Drawing for the job (mm, zero at the part's lowest x, y, z). A direction names the side the tool comes from. Round coordinates to 2 decimals unless told otherwise and drop trailing zeros. Write each loop counter-clockwise with the first axis right and the second up, starting at its lowest first coordinate (ties: lowest second). Pieces come first, ordered by that corner, then holes.
Item 1: Band-saw the part on D-D, the plane z = 36. Write the cut outline in (x, y).
Item 2: Band-saw the part on B-B, the plane z = 9. Write the cut outline in (x, y).
Item 3: Band-saw the part on C-C, the plane y = 2.5. Count the separate pieces of the cut face and the enclosed holes in it, then the cut area to 3 significant figures.
Item 4: 3-axis set-ups, long thin cutter, end or side, ignore diameter. For the marked faces 5, 6 and 7: which of +Z, -Z, +X, -X, +Y, -Y reach the whole face in a straight line?
Item 5: Mould opens along X. For the marked faces 1, 2, 3 and 4 say: +X half, -X half, draft (parallel to the pull), parting line (faces both ways), or undercut.
Item 6: Wall check: probe 1 along Y at (x, z) = (18.5, 36.5); probe 2 along X at (y, z) = (3, 14.5) (1 decimal); probe 3 along X at (y, z) = (3.25, 19.5) (1 decimal). Give the ranges that are in metal, low to high.
Item 7: Band-saw the part on A-A, the plane z = 4.5. Write the cut outline in (x, y) (1 decimal), then the cut area to 3 significant figures.
Item 8: Drop flat-ended pins along their axis: pin 1 Ø1.2 at (x, y) = (23, 2.5) entering from -Z; pin 2 Ø4 at (y, z) = (5, 34.5) entering from +X; pin 3 Ø3 at (x, z) = (4.62, 4.83) entering from -Y; pin 4 Ø3 at (y, z) = (3, 14.5) entering from -X. Give the stop position or say it passes through.
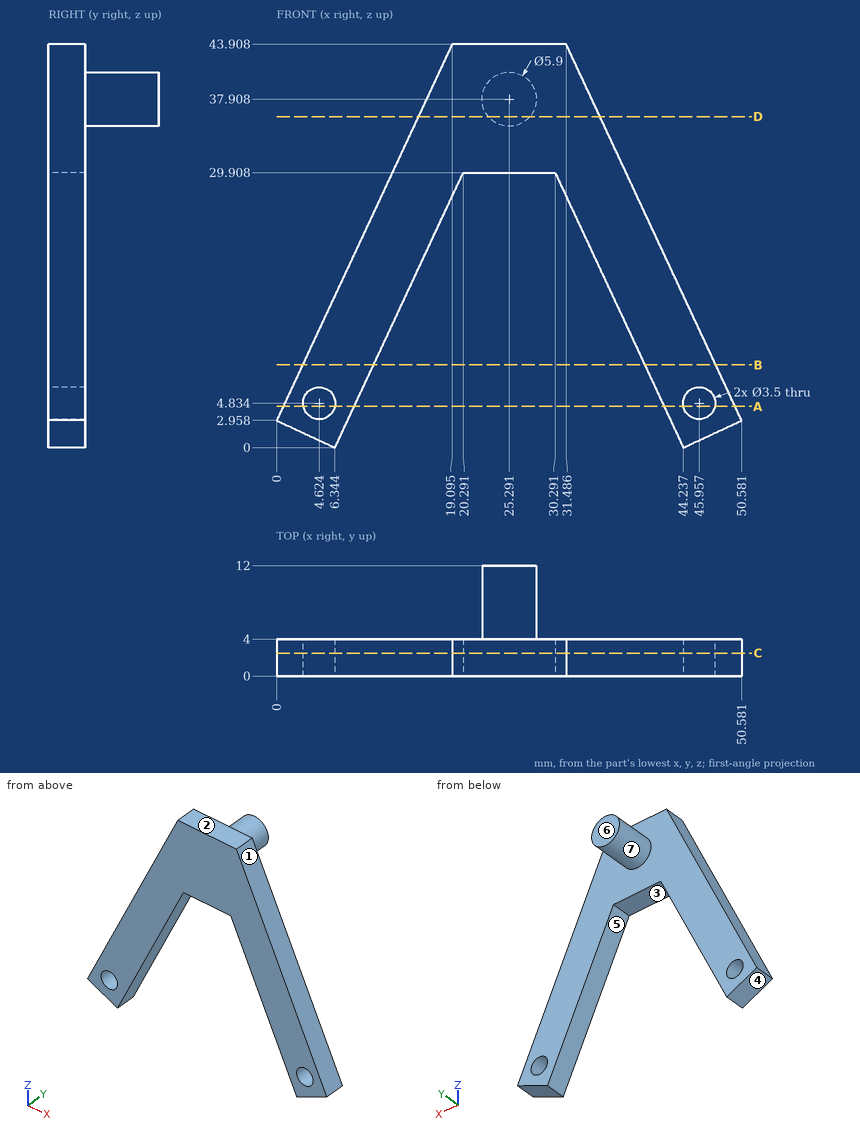
Results:
1. outline: (15.41, 0) - (35.17, 0) - (35.17, 4) - (27.54, 4) - (27.54, 12) - (23.04, 12) - (23.04, 4) - (15.41, 4) - close
2. outline: (2.82, 0) - (10.54, 0) - (10.54, 4) - (2.82, 4) - close; (40.04, 0) - (47.76, 0) - (47.76, 4) - (40.04, 4) - close
3. separate pieces: 1
3. enclosed holes: 2
3. area: 685 mm2
4. face 5: -Z, +Y, -Y
4. face 6: +Z, -Z, +X, -X, +Y
4. face 7: +Y
5. face 1: +X half
5. face 2: draft
5. face 3: undercut
5. face 4: -X half
6. probe 1: y = 0 to 4
6. probe 2: x = 5.4 to 13.1, 37.5 to 45.2
6. probe 3: x = 7.7 to 15.4, 35.1 to 42.9
7. outline: (0.7, 0) - (2.9, 0) - (2.9, 4) - (0.7, 4) - close; (6.3, 0) - (8.4, 0) - (8.4, 4) - (6.3, 4) - close; (42.1, 0) - (44.2, 0) - (44.2, 4) - (42.1, 4) - close; (47.7, 0) - (49.9, 0) - (49.9, 4) - (47.7, 4) - close
7. area: 34.3 mm2
8. pin 1: stops at z = 29.91
8. pin 2: stops at x = 36.68
8. pin 3: passes through
8. pin 4: stops at x = 4.68
